Could you check a few things on this drawing? It's one solid part, dimensions in mm from its lowest x, y, z. A direction names the side the tool comes from. Round coordinates to 2 decimals unless told otherwise and drop trailing zeros. Write each loop counter-clockwise with the first axis right and the second up, starting at its lowest first coordinate (ties: lowest second). Pieces come first, ordered by that corner, then holes. Notation, with made-up numbers: (47, 10.25) -> (63, 10.25) arc R23 cw to (63, 43.25) -> close; hole circle Ø5 at (-20, -24). An arc over 180 degrees is marked (long way). Return JSON: item names as keys, results as strings.
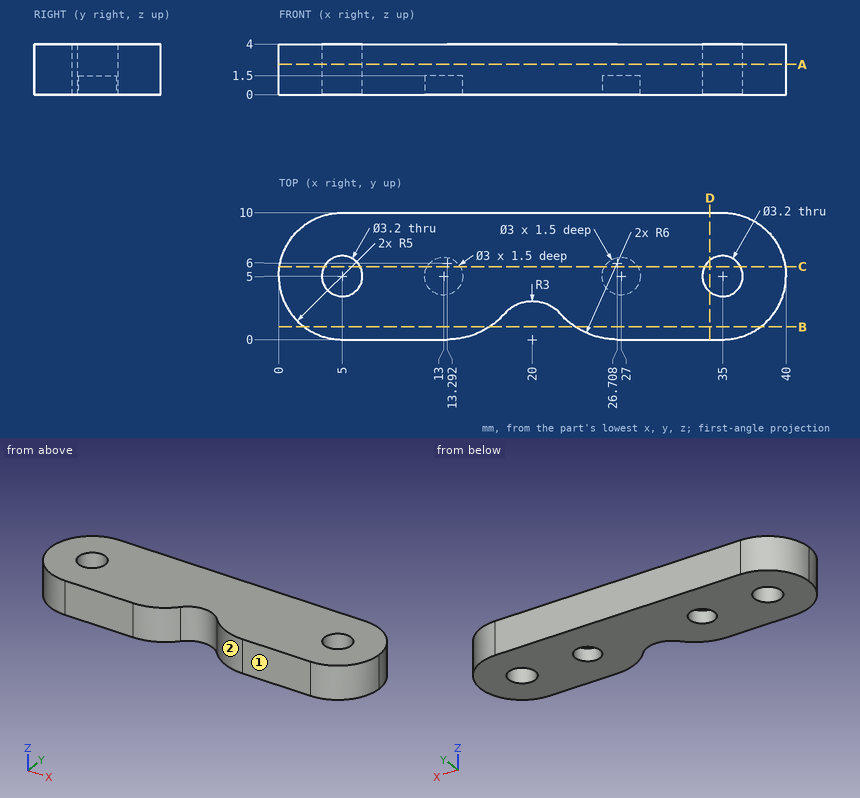
1) I want a section at A-A, the plane z = 2.4. Count the separate pieces of the cut face and the enclosed holes in it, and give its area (3 significant figures).
Return value:
{"separate pieces": "1", "enclosed holes": "2", "area": "345 mm²"}
2) I want a section at D-D, the plane x = 34. Please give me the cut outline in (y, z).
Return value:
{"outline": "(0, 0) -> (3.75, 0) -> (3.75, 4) -> (0, 4) -> close; (6.25, 0) -> (10, 0) -> (10, 4) -> (6.25, 4) -> close"}
3) Will these pins go through, and if not, where does the flat tip stop? pin 1 Ø1 at (y, z) = (1.5, 1.5) entering from +X; pin 2 Ø0.9 at (x, y) = (26.5, 5) entering from -Z; pin 3 Ø2 at (x, z) = (22, 3.5) entering from -Y; pin 4 Ø1.5 at (y, z) = (5.5, 2) entering from -X.
Return value:
{"pin 1": "x = 39", "pin 2": "z = 1.5", "pin 3": "y = 1.28", "pin 4": "x = 0"}
4) I want a section at C-C, the plane y = 5.75. Please give me the cut outline in (x, z), and give its area (3 significant figures).
Return value:
{"outline": "(0.06, 0) -> (3.59, 0) -> (3.59, 4) -> (0.06, 4) -> close; (6.41, 0) -> (11.7, 0) -> (11.7, 1.5) -> (14.3, 1.5) -> (14.3, 0) -> (25.7, 0) -> (25.7, 1.5) -> (28.3, 1.5) -> (28.3, 0) -> (33.59, 0) -> (33.59, 4) -> (6.41, 4) -> close; (36.41, 0) -> (39.94, 0) -> (39.94, 4) -> (36.41, 4) -> close", "area": "129 mm²"}
5) For the marked faces 1 and 2, which set-ups out of +Z, -Z, +X, -X, +Y, -Y let a thin tool reach every point of the face, with its end or its side?
Return value:
{"face 1": "+Z, -Z, +X, -X, -Y", "face 2": "+Z, -Z, -Y"}
6) I want a section at B-B, the plane y = 1. Please give me the cut outline in (x, z), and give its area (3 significant figures).
Return value:
{"outline": "(2, 0) -> (16.61, 0) -> (16.61, 4) -> (2, 4) -> close; (23.39, 0) -> (38, 0) -> (38, 4) -> (23.39, 4) -> close", "area": "117 mm²"}
7) If I drill on probe 1 along Y at (x, z) = (13, 1); probe 2 along Y at (x, z) = (35, 2.4); probe 3 along X at (y, z) = (3.75, 0.25), over which ranges is the centre line in solid material (lowest first)? Write a range as [from, to].
Return value:
{"probe 1": "[0, 3.5], [6.5, 10]", "probe 2": "[0, 3.4], [6.6, 10]", "probe 3": "[0.16, 4], [6, 12.17], [13.83, 26.17], [27.83, 34], [36, 39.84]"}
